CAD build for the part. Positions are in the model's coordinates, mm. A direction names the side the tool comes from. Round coordinates to 2 decimals unless told otherwise and drop trailing zeros. Order: outer loops, then holes, each group sorted by start corner. A loop starts at its lowest first (then second) coordinate and runs counter-clockwise, first axis right, second up. Notation, with made-up numbers: (-6, 12) - (46, 12) arc R9 ccw to (46, 29) - close; hole circle Ø2 at (38, -29.75). An arc over 180 degrees is marked (long way). Write item = value, one per line.
from build123d import *

# Parameters (mm, degrees)
SKETCH1_R             = 2.286
SKETCH1_R_2           = 11.1125
SKETCH1_R_3           = 7.366
BOSS_EXTRUDE1_DEPTH   = 16.51
SKETCH2_R             = 12.7
CUT_EXTRUDE1_DEPTH    = 1.778
CAVITY1_START         = 5.334
CAVITY1_OUTLINE_R     = 1.143
CAVITY1_OUTLINE_R_2   = 7.366
CAVITY1_OUTLINE_R_3   = 4.445
CAVITY1_DEPTH         = 11.176
CAVITY1_START_2       = 15.494
CAVITY1_2_OUTLINE_R   = 1.143
CAVITY1_2_OUTLINE_R_2 = 4.445
CAVITY1_2_DEPTH       = 1.016
CAVITY1_START_3       = 2.286
CAVITY1_3_OUTLINE_R   = 1.143
CAVITY1_3_OUTLINE_R_2 = 4.445
CAVITY1_3_DEPTH       = 3.048
CAVITY1_4_OUTLINE_R   = 1.905
CAVITY1_4_DEPTH       = 3.302
CAVITY1_START_4       = 13.716
CAVITY1_5_DEPTH       = 1.778
CAVITY1_START_5       = 4.064
CAVITY1_6_OUTLINE_R   = 2.286
CAVITY1_6_DEPTH       = 1.27
CAVITY1_START_6       = 2.032
CAVITY1_7_DEPTH       = 0.254
FILLET1_R             = 2.54


# Read off the part's stored shape, not the designer's step: Cavity1
with BuildPart() as part:
    # Sketch1 → Boss-Extrude1 (new body)
    with BuildSketch(Plane.XY):
        with BuildLine():
            Line((-6.35, 19.05), (6.35, 19.05))
            Line((6.35, 19.05), (6.35, -38.1))
            Line((6.35, -38.1), (14.999447267, -86.202930908))
            ThreePointArc((14.999447267, -86.202930908), (5.413612396, -103.146066153), (-13.00522541, -96.844917372))
            Line((-13.00522541, -96.844917372), (-41.91, -49.53))
            Line((-41.91, -49.53), (-41.91, 11.43))
            Line((-41.91, 11.43), (-6.35, 19.05))
        make_face()
        with Locations((0, 12.7)):
            Circle(SKETCH1_R, mode=Mode.SUBTRACT)
        with Locations(Location((0, -12.7, 0), (0, 0, 180))):
            Circle(SKETCH1_R, mode=Mode.SUBTRACT)
        with Locations((0, -88.9)):
            Circle(SKETCH1_R_2, mode=Mode.SUBTRACT)
        with Locations((-24.13, -7.62)):
            Circle(SKETCH1_R_3, mode=Mode.SUBTRACT)
    extrude(amount=BOSS_EXTRUDE1_DEPTH)

    # Sketch2 → Cut-Extrude1 (cut)
    with BuildSketch(Plane(origin=(0, 0, 0), x_dir=(-1, 0, 0), z_dir=(0, 0, -1))):
        with Locations((0, -88.9)):
            Circle(SKETCH2_R)
    extrude(amount=-CUT_EXTRUDE1_DEPTH, mode=Mode.SUBTRACT)

    # Cavity1 outline → Cavity1 (cut)
    # profile 1 of 6: a face of its own
    with BuildSketch(Plane.XY.offset(CAVITY1_START)):
        with Locations((-38.1, 1.524)):
            Circle(CAVITY1_OUTLINE_R)
    # profile 2 of 6: a face of its own
    with BuildSketch(Plane.XY.offset(CAVITY1_START)):
        with BuildLine():
            ThreePointArc((-34.194128852, 2.610567504), (-38.481, -7.62), (-34.194128852, -17.850567504))
            ThreePointArc((-34.194128852, -17.850567504), (-34.366847552, -21.659105214), (-30.793505747, -20.330188518))
            ThreePointArc((-30.793505747, -20.330188518), (-24.13, -21.971), (-17.466494253, -20.330188518))
            ThreePointArc((-17.466494253, -20.330188518), (-13.893152448, -21.659105214), (-14.065871148, -17.850567504))
            ThreePointArc((-14.065871148, -17.850567504), (-9.779, -7.62), (-14.065871148, 2.610567504))
            ThreePointArc((-14.065871148, 2.610567504), (-13.893152448, 6.419105214), (-17.466494253, 5.090188518))
            ThreePointArc((-17.466494253, 5.090188518), (-24.13, 6.731), (-30.793505747, 5.090188518))
            ThreePointArc((-30.793505747, 5.090188518), (-34.366847552, 6.419105214), (-34.194128852, 2.610567504))
        make_face()
        with Locations((-24.13, -7.62)):
            Circle(CAVITY1_OUTLINE_R_2, mode=Mode.SUBTRACT)
    # profile 3 of 6: a face of its own
    with BuildSketch(Plane.XY.offset(CAVITY1_START)):
        with Locations((-38.1, -42.164)):
            Circle(CAVITY1_OUTLINE_R)
    # profile 4 of 6: a face of its own
    with BuildSketch(Plane.XY.offset(CAVITY1_START)):
        with Locations((-24.13, -33.02)):
            Circle(CAVITY1_OUTLINE_R_3)
    # profile 5 of 6: a face of its own
    with BuildSketch(Plane.XY.offset(CAVITY1_START)):
        with Locations((-10.16, 1.524)):
            Circle(CAVITY1_OUTLINE_R)
    # profile 6 of 6: a face of its own
    with BuildSketch(Plane.XY.offset(CAVITY1_START)):
        with Locations((-10.16, -42.164)):
            Circle(CAVITY1_OUTLINE_R)
    extrude(amount=CAVITY1_DEPTH, mode=Mode.SUBTRACT)

    # Cavity1 2 outline → Cavity1 2 (cut)
    with BuildSketch(Plane.XY.offset(CAVITY1_START_2)):
        with BuildLine():
            ThreePointArc((-40.767, -45.593), (-39.725471714, -48.107471714), (-37.211, -49.149))
            Line((-37.211, -49.149), (-11.049, -49.149))
            ThreePointArc((-11.049, -49.149), (-8.534528286, -48.107471714), (-7.493, -45.593))
            Line((-7.493, -45.593), (-7.493, 4.953))
            ThreePointArc((-7.493, 4.953), (-8.534528286, 7.467471714), (-11.049, 8.509))
            Line((-11.049, 8.509), (-37.211, 8.509))
            ThreePointArc((-37.211, 8.509), (-39.725471714, 7.467471714), (-40.767, 4.953))
            Line((-40.767, 4.953), (-40.767, -45.593))
        make_face()
        with Locations((-38.1, 1.524)):
            Circle(CAVITY1_2_OUTLINE_R, mode=Mode.SUBTRACT)
        with BuildLine():
            ThreePointArc((-34.194128852, 2.610567504), (-34.366847552, 6.419105214), (-30.793505747, 5.090188518))
            ThreePointArc((-30.793505747, 5.090188518), (-24.13, 6.731), (-17.466494253, 5.090188518))
            ThreePointArc((-17.466494253, 5.090188518), (-13.893152448, 6.419105214), (-14.065871148, 2.610567504))
            ThreePointArc((-14.065871148, 2.610567504), (-9.779, -7.62), (-14.065871148, -17.850567504))
            ThreePointArc((-14.065871148, -17.850567504), (-13.893152448, -21.659105214), (-17.466494253, -20.330188518))
            ThreePointArc((-17.466494253, -20.330188518), (-24.13, -21.971), (-30.793505747, -20.330188518))
            ThreePointArc((-30.793505747, -20.330188518), (-34.366847552, -21.659105214), (-34.194128852, -17.850567504))
            ThreePointArc((-34.194128852, -17.850567504), (-38.481, -7.62), (-34.194128852, 2.610567504))
        make_face(mode=Mode.SUBTRACT)
        with Locations((-24.13, -33.02)):
            Circle(CAVITY1_2_OUTLINE_R_2, mode=Mode.SUBTRACT)
        with Locations((-38.1, -42.164)):
            Circle(CAVITY1_2_OUTLINE_R, mode=Mode.SUBTRACT)
        with Locations((-10.16, 1.524)):
            Circle(CAVITY1_2_OUTLINE_R, mode=Mode.SUBTRACT)
        with Locations((-10.16, -42.164)):
            Circle(CAVITY1_2_OUTLINE_R, mode=Mode.SUBTRACT)
    extrude(amount=CAVITY1_2_DEPTH, mode=Mode.SUBTRACT)

    # Cavity1 3 outline → Cavity1 3 (cut)
    with BuildSketch(Plane.XY.offset(CAVITY1_START_3)):
        with Locations((-38.1, 1.524)):
            Circle(CAVITY1_3_OUTLINE_R)
        with Locations((-38.1, -42.164)):
            Circle(CAVITY1_3_OUTLINE_R)
        with BuildLine():
            ThreePointArc((-20.50956216, -21.506815), (-24.13, -16.51), (-27.75043784, -21.506815))
            ThreePointArc((-27.75043784, -21.506815), (-24.13, -21.971), (-20.50956216, -21.506815))
        make_face()
        with Locations((-24.13, -33.02)):
            Circle(CAVITY1_3_OUTLINE_R_2)
        with Locations((-10.16, 1.524)):
            Circle(CAVITY1_3_OUTLINE_R)
        with Locations((-10.16, -42.164)):
            Circle(CAVITY1_3_OUTLINE_R)
    extrude(amount=CAVITY1_3_DEPTH, mode=Mode.SUBTRACT)

    # Cavity1 4 outline → Cavity1 4 (cut)
    with BuildSketch(Plane.XY):
        with Locations((-38.1, 1.524)):
            Circle(CAVITY1_4_OUTLINE_R)
        with Locations((-38.1, -42.164)):
            Circle(CAVITY1_4_OUTLINE_R)
        with Locations((-10.16, 1.524)):
            Circle(CAVITY1_4_OUTLINE_R)
        with Locations((-10.16, -42.164)):
            Circle(CAVITY1_4_OUTLINE_R)
    extrude(amount=CAVITY1_4_DEPTH, mode=Mode.SUBTRACT)

    # Cavity1 5 outline → Cavity1 5 (cut)
    with BuildSketch(Plane.XY.offset(CAVITY1_START_4)):
        with BuildLine():
            Line((-28.458512749, -32.009058667), (-30.399761763, -33.918725966))
            ThreePointArc((-30.399761763, -33.918725966), (-29.735544051, -37.908349777), (-26.797234263, -40.687669641))
            Line((-26.797234263, -40.687669641), (-25.65265334, -37.196068942))
            ThreePointArc((-25.65265334, -37.196068942), (-28.039642573, -35.1348806), (-28.458512749, -32.009058667))
        make_face()
        with BuildLine():
            ThreePointArc((-25.391900971, -28.701648336), (-28.711043619, -30.52766679), (-30.399761763, -33.918725966))
            Line((-30.399761763, -33.918725966), (-28.458512749, -32.009058667))
            ThreePointArc((-28.458512749, -32.009058667), (-27.357510815, -29.963662495), (-25.375086436, -28.752941907))
            Line((-25.375086436, -28.752941907), (-25.391900971, -28.701648336))
        make_face()
        with BuildLine():
            ThreePointArc((-25.033307826, -28.639577582), (-25.213049158, -28.66804351), (-25.391900971, -28.701648336))
            Line((-25.391900971, -28.701648336), (-25.375086436, -28.752941907))
            ThreePointArc((-25.375086436, -28.752941907), (-25.223135952, -28.711510846), (-25.069813075, -28.675488936))
            Line((-25.069813075, -28.675488936), (-25.033307826, -28.639577582))
        make_face()
        with BuildLine():
            Line((-25.65265334, -37.196068942), (-26.797234263, -40.687669641))
            ThreePointArc((-26.797234263, -40.687669641), (-24.13, -41.275), (-21.462765737, -40.687669641))
            Line((-21.462765737, -40.687669641), (-22.60734666, -37.196068942))
            ThreePointArc((-22.60734666, -37.196068942), (-24.13, -37.465), (-25.65265334, -37.196068942))
        make_face()
        with BuildLine():
            Line((-23.190186925, -28.675488936), (-23.226692174, -28.639577582))
            ThreePointArc((-23.226692174, -28.639577582), (-23.67719342, -28.591164969), (-24.130000054, -28.575))
            ThreePointArc((-24.130000054, -28.575), (-23.657414944, -28.600193628), (-23.190186925, -28.675488936))
        make_face()
        with BuildLine():
            ThreePointArc((-22.868099029, -28.701648336), (-23.046950842, -28.66804351), (-23.226692174, -28.639577582))
            Line((-23.226692174, -28.639577582), (-23.190186925, -28.675488936))
            ThreePointArc((-23.190186925, -28.675488936), (-23.036864049, -28.711510846), (-22.884913564, -28.752941907))
            Line((-22.884913564, -28.752941907), (-22.868099029, -28.701648336))
        make_face()
        with BuildLine():
            ThreePointArc((-24.130000054, -28.575), (-24.582806633, -28.591164973), (-25.033307826, -28.639577582))
            Line((-25.033307826, -28.639577582), (-25.069813075, -28.675488936))
            ThreePointArc((-25.069813075, -28.675488936), (-24.60258511, -28.600193634), (-24.130000054, -28.575))
        make_face()
        with BuildLine():
            Line((-22.60734666, -37.196068942), (-21.462765737, -40.687669641))
            ThreePointArc((-21.462765737, -40.687669641), (-18.77932539, -38.344470897), (-17.78, -34.925))
            ThreePointArc((-17.78, -34.925), (-17.800091344, -34.420266009), (-17.860238237, -33.918725967))
            Line((-17.860238237, -33.918725967), (-19.80148725, -32.009058668))
            ThreePointArc((-19.80148725, -32.009058668), (-19.71421784, -32.511184794), (-19.685, -33.02))
            ThreePointArc((-19.685, -33.02), (-20.488144766, -35.5685124), (-22.60734666, -37.196068942))
        make_face()
        with BuildLine():
            ThreePointArc((-17.860238237, -33.918725967), (-19.548956381, -30.52766679), (-22.868099029, -28.701648336))
            Line((-22.868099029, -28.701648336), (-22.884913564, -28.752941907))
            ThreePointArc((-22.884913564, -28.752941907), (-20.902489185, -29.963662496), (-19.80148725, -32.009058668))
            Line((-19.80148725, -32.009058668), (-17.860238237, -33.918725967))
        make_face()
    extrude(amount=CAVITY1_5_DEPTH, mode=Mode.SUBTRACT)

    # Cavity1 6 outline → Cavity1 6 (cut)
    with BuildSketch(Plane.XY.offset(CAVITY1_START_5)):
        with Locations((-33.02, 4.572)):
            Circle(CAVITY1_6_OUTLINE_R)
        with Locations((-33.02, -19.812)):
            Circle(CAVITY1_6_OUTLINE_R)
        with Locations((-15.24, 4.572)):
            Circle(CAVITY1_6_OUTLINE_R)
        with Locations((-15.24, -19.812)):
            Circle(CAVITY1_6_OUTLINE_R)
    extrude(amount=CAVITY1_6_DEPTH, mode=Mode.SUBTRACT)

    # Cavity1 7 outline → Cavity1 7 (cut)
    with BuildSketch(Plane.XY.offset(CAVITY1_START_6)):
        with BuildLine():
            ThreePointArc((-20.50956216, -21.506815), (-24.13, -16.51), (-27.75043784, -21.506815))
            ThreePointArc((-27.75043784, -21.506815), (-24.13, -21.971), (-20.50956216, -21.506815))
        make_face()
    extrude(amount=CAVITY1_7_DEPTH, mode=Mode.SUBTRACT)

    # Fillet1
    fillet1_edges = [part.edges().sort_by_distance(p)[0] for p in [
        (6.35, -38.1, 8.255),
        (-41.91, -49.53, 8.255),
        (-41.91, 11.43, 8.255),
        (-6.35, 19.05, 8.255),
        (6.35, 19.05, 8.255),
    ]]
    fillet(fillet1_edges, radius=FILLET1_R)


solid = part.part
(1) Band-saw the part on D-D on x = -15.24. List the corners of the cut face in (y, z) (3 decimals).
Solved:
outline = (-93.187, 0) - (17.145, 0) - (17.145, 16.51) - (8.509, 16.51) - (8.509, 15.494) - (6.858, 15.494) - (6.858, 4.064) - (2.286, 4.064) - (2.286, 5.334) - (-17.526, 5.334) - (-17.526, 4.064) - (-22.098, 4.064) - (-22.098, 15.494) - (-49.149, 15.494) - (-49.149, 16.51) - (-93.187, 16.51) - close
(2) Pull direction X, two halves, no side cores. Call faces 4 (the cylindrical face through (5.586, 18.326, 8.371)), 5 (the cylindrical face through (-40.003, 1.608, 1.628)): released by +X, released by -X, zero draft, split by the parting line, or undercut.
Solved:
face_4 = released by +X
face_5 = undercut
(3) Drop flat-ended pins along their axis: pin 1 (20.5 mm diameter, centred on x = 4, y = -92.5, fed in from -Z); pin 2 (2.5 mm diameter, centred on x = -38.1, y = 1.524, fed in from -Z); pin 3 (0.8 mm diameter, centred on x = -27.5, z = 16, fed in from +Y); pin 4 (4 mm diameter, centred on x = 0, y = -12.7, fed in from +Z). Give the stop position or say it passes through.
Solved:
pin_1 = 0
pin_2 = 3.3
pin_3 = 14.6
pin_4 = through
(4) Tool access for faces 1 (the flat face through (-9, -43, 3.302)), 2 (the cylindrical face through (1.229, 14.628, 8.139)), 3 (the cylindrical face through (-39.75, -48.08, 15.99)): list every direction of +Z, -Z, +X, -X, +Y, -Y with a clear straight run to the whole face (end or side of a thin tool).
Solved:
face_1 = -Z
face_2 = +Z, -Z
face_3 = +Z
(5) Probe line 1 along Y through (x, z) = (-24.13, 9.5) (1 decimal); line 2 along Y through (x, z) = (-22, 3); line 3 along Y through (x, z) = (-38.1, 1.1). List the from-to ranges inside material, lowest first.
Solved:
line_1 = -78.6 to -37.5, -28.6 to -22, 6.7 to 15.2
line_2 = -82.12 to -36.92, -29.12 to -21.81, -17.16 to -14.67, -0.57 to 15.7
line_3 = -55.77 to -44.07, -40.26 to -0.38, 3.43 to 12.25
(6) Band-saw the part on C-C on z = 11.75. Count the separate pieces of the cut face and the enclosed holes in it, plus the area to 3 significant figures.
Solved:
separate_pieces = 1
enclosed_holes = 9
area = 4,010 mm²
(7) Band-saw the part on A-A on x = 0. List the corners of the cut face in (y, z).
Solved:
outline = (-104.14, 0) - (-101.6, 0) - (-101.6, 1.78) - (-100.01, 1.78) - (-100.01, 16.51) - (-104.14, 16.51) - close; (-77.79, 1.78) - (-76.2, 1.78) - (-76.2, 0) - (-14.99, 0) - (-14.99, 16.51) - (-77.79, 16.51) - close; (-10.41, 0) - (10.41, 0) - (10.41, 16.51) - (-10.41, 16.51) - close; (14.99, 0) - (19.05, 0) - (19.05, 16.51) - (14.99, 16.51) - close
(8) Band-saw the part on B-B on y = -12.7. List the corners of the cut face in (x, z).
Solved:
outline = (-41.91, 0) - (-29.46, 0) - (-29.46, 5.33) - (-37.55, 5.33) - (-37.55, 15.49) - (-40.77, 15.49) - (-40.77, 16.51) - (-41.91, 16.51) - close; (-18.8, 0) - (-2.29, 0) - (-2.29, 16.51) - (-7.49, 16.51) - (-7.49, 15.49) - (-10.71, 15.49) - (-10.71, 5.33) - (-18.8, 5.33) - close; (2.29, 0) - (6.35, 0) - (6.35, 16.51) - (2.29, 16.51) - close
